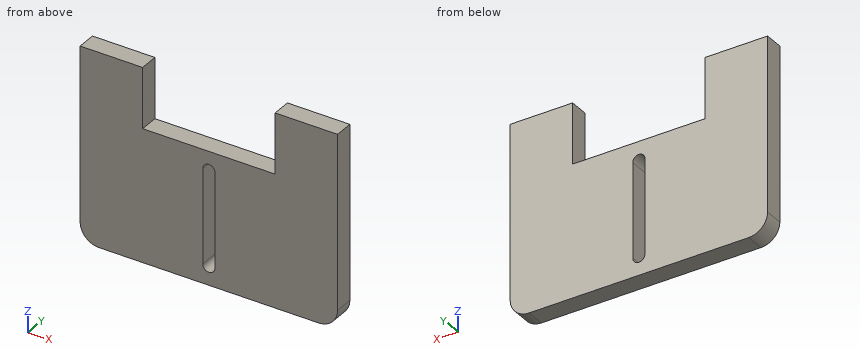
from build123d import *

# Parameters (mm, degrees)
EXTRUDE_1_DEPTH = 5
SKETCH_2_W      = 4
SKETCH_2_H      = 28
EXTRUDE_2_DEPTH = 5
FILLET_1_R      = 5


with BuildPart() as part:
    # 草图1 → 凸台-拉伸1 (new body)
    with BuildSketch(Plane(origin=(0, 0, 0), x_dir=(1, 0, 0), z_dir=(0, 1, 0))):
        Polygon((30, 22.84905584), (-30, 22.84905584), (-30, -5.15094416), (-34, -5.15094416), (-34, -28.15094416), (-17.5, -28.15094416), (-17.5, -12.15094416), (17.5, -12.15094416), (17.5, -28.15094416), (34, -28.15094416), (34, -5.15094416), (30, -5.15094416), align=None)
        with BuildLine():
            Line((1.6, 17.84905584), (1.6, -7.15094416))
            ThreePointArc((1.6, -7.15094416), (0, -8.75094416), (-1.6, -7.15094416))
            Line((-1.6, -7.15094416), (-1.6, 17.84905584))
            ThreePointArc((-1.6, 17.84905584), (0, 19.44905584), (1.6, 17.84905584))
        make_face(mode=Mode.SUBTRACT)
    extrude(amount=EXTRUDE_1_DEPTH)

    # 草图2 → 凸台-拉伸2 (add)
    with BuildSketch(Plane(origin=(0, 0, 0), x_dir=(1, 0, 0), z_dir=(0, 1, 0))):
        with Locations((-32, 8.84905584)):
            Rectangle(SKETCH_2_W, SKETCH_2_H)
        with Locations((32, 8.84905584)):
            Rectangle(SKETCH_2_W, SKETCH_2_H)
    extrude(amount=EXTRUDE_2_DEPTH)

    # 圆角1
    fillet_1_edges = [part.edges().sort_by_distance(p)[0] for p in [
        (-34, 2.5, -22.84905584),
        (34, 2.5, -22.84905584),
    ]]
    fillet(fillet_1_edges, radius=FILLET_1_R)


solid = part.part
The model under review builds one solid part; all positions refer to its coordinate system, in mm. Round coordinates to 2 decimals unless told otherwise and drop trailing zeros. Write each loop counter-clockwise with the first axis right and the second up, starting at its lowest first coordinate (ties: lowest second). Pieces come first, ordered by that corner, then holes. Notation, with made-up numbers: M 37.5,32 L 61.5,32 A26 ccw 61.5,69 Z; hole C 29,57.5 d11. An arc over 180 degrees is marked long. Use a Markdown table: item, result. Add a question column.
Q1. We need section C-C, the plane y = 2.75. State the section outline as (x, z) points, plus the area to 3 significant figures.
Q2. To check wall thickness, follow line 1 (X direction, y = 1.3, z = -10); line 2 (X direction, y = 2.3, z = 23.5); line 3 (Z direction, x = 14, y = 3.9). State the ranges of each line that lie inside material, in increasing order.
Q3. We need section B-B, the plane z = -7.5. State the section outline as (x, y) points.
Q4. We need section A-A, the plane x = 0. State the section outline as (y, z) points, plus the area to 3 significant figures.
Q5. Insertion check: pin 1 (2.5 mm diameter, centred on x = -6.5, y = 2, fed in from +Z); pin 2 (8 mm diameter, centred on x = 10, z = 20.5, fed in from -Y); pin 3 (4 mm diameter, centred on x = 20, z = 21.5, fed in from -Y). Each pin has a flat end and moves straight along its axis. Give the tip position at first contact, or say it passes through.
Findings below:
| question | item | result |
|---|---|---|
| 1 | outline | M -34,-17.85 A5 ccw -29,-22.85 L 29,-22.85 A5 ccw 34,-17.85 L 34,28.15 L 17.5,28.15 L 17.5,12.15 L -17.5,12.15 L -17.5,28.15 L -34,28.15 Z; hole M -1.6,-17.85 A1.6 ccw 1.6,-17.85 L 1.6,7.15 A1.6 ccw -1.6,7.15 Z |
| 1 | area | 2,810 mm² |
| 2 | line 1 | x = -34 to -1.6, 1.6 to 34 |
| 2 | line 2 | x = -34 to -17.5, 17.5 to 34 |
| 2 | line 3 | z = -22.85 to 12.15 |
| 3 | outline | M -34,0 L -1.6,0 L -1.6,5 L -34,5 Z; M 1.6,0 L 34,0 L 34,5 L 1.6,5 Z |
| 4 | outline | M 0,-22.85 L 5,-22.85 L 5,-19.45 L 0,-19.45 Z; M 0,8.75 L 5,8.75 L 5,12.15 L 0,12.15 Z |
| 4 | area | 34.0 mm² |
| 5 | pin 1 | stops at z = 12.15 |
| 5 | pin 2 | passes through |
| 5 | pin 3 | stops at y = 0 |
